Input: part model. Units: mm. Frame: model coordinates. A direction names the side the tool comes from. Round coordinates to 2 decimals unless told otherwise and drop trailing zeros. Order: outer loops, then holes, each group sorted by start corner. A loop starts at its lowest first (then second) coordinate and runs counter-clockwise, first axis right, second up.
Item 1: Cut plane A-A on z = 30.5. Output: boundary loops of the cut face in (x, y).
Item 2: Line query: L1, parallel to Y at x = 56, z = -65; L2, parallel to Y at x = 30, z = 36.5; L3, parallel to X at y = -20, z = 40.5. Output: solid intervals per line, ascending.
Item 3: Cut plane C-C on y = -24.5. Output: boundary loops of the cut face in (x, z), then the cut area to 3 significant figures.
Item 4: Reachability of faces 1 (the cylindrical face through (33.087, 12.325, 49.192)), 2 (the flat face through (-1.544, -14, 40)), 3 (the flat face through (-16, 0, -23)), 4 (the flat face through (36.48, -25.35, 28.87)) from +Z, -Z, +X, -X, +Y, -Y: full face, straight path, thin tool, end or side. Return the list, or none.
Item 5: First-contact query: pin 1 (4 mm diameter, centred on x = -10.5, z = 25.5, fed in from +Y); pin 2 (1 mm diameter, centred on y = -5, z = 15.5, fed in from +X). Flat tips, straight axial feed; report the tip coordinate or a pass-through.
Item 6: Cut plane B-B on x = 21.5. Output: boundary loops of the cut face in (y, z), then the cut area to 3 significant figures.
Item 7: Cut plane D-D on x = 54. Output: boundary loops of the cut face in (y, z), then the cut area to 3 significant figures.
```python
from build123d import *

# Parameters (mm, degrees)
F0_W     = 144.018009305
F0_H     = 126.3136602938
F1_DEPTH = 50
F3_DEPTH = 75
F4_R     = 23.2012812913
F5_DEPTH = 25


with BuildPart() as f1:
    # F0 (on Front) → F1 (new body)
    with BuildSketch(Plane.XZ):
        with Locations((1.4469921589, -9.7884591669)):
            Rectangle(F0_W, F0_H)
    extrude(amount=F1_DEPTH)

    # F2 (on face) → F3 (cut)
    with BuildSketch(Plane.YZ.offset(73.4559968114)):
        Polygon((0, 53.36837098), (-50, 53.36837098), (0, 3.6792913452), align=None)
    extrude(amount=-F3_DEPTH, mode=Mode.SUBTRACT)

    # F4 (on face) → F5 (join)
    with BuildSketch(Plane.XZ):
        with Locations((36.1069515347, 26.1881500483)):
            Circle(F4_R)
    extrude(amount=-F5_DEPTH)


solid = f1.part
```
From the geometry:
1. outline: (-70.56, -50) - (73.46, -50) - (73.46, -26.99) - (-1.54, -26.99) - (-1.54, 0) - (-70.56, 0) - close; (13.31, 0) - (58.9, 0) - (58.9, 25) - (13.31, 25) - close
2. L1: y = -50 to 0
2. L2: y = -50 to -33.03, 0 to 25
2. L3: x = -70.56 to -1.54
3. outline: (-70.56, -72.95) - (73.46, -72.95) - (73.46, 28.03) - (-1.54, 28.03) - (-1.54, 53.37) - (-70.56, 53.37) - close
3. area: 16,300 mm2
4. face 1: +Y
4. face 2: +Z, +X, +Y
4. face 3: -Z, -X, +Y
4. face 4: +Z, +X
5. pin 1: stops at y = 0
5. pin 2: stops at x = -1.54
6. outline: (-50, -72.95) - (0, -72.95) - (0, 3.68) - (-50, 53.37) - close; (0, 8.16) - (25, 8.16) - (25, 44.21) - (0, 44.21) - close
6. area: 5,970 mm2
7. outline: (-50, -72.95) - (0, -72.95) - (0, 3.68) - (-50, 53.37) - close; (0, 11.42) - (25, 11.42) - (25, 40.96) - (0, 40.96) - close
7. area: 5,810 mm2
